Check sheet for the drawn part. Datum: minimum x, y, z corner. Units: mm. Coordinates: 2 decimals unless noted, no trailing zeros. Loops run counter-clockwise (first coordinate to the right, second up) from the corner with the lowest first, then second, coordinate; pieces in that order, holes last. Notation, with made-up numbers: (19, 14) -> (78, 14) arc R23 ccw to (78, 43) -> close; hole circle Ø5 at (85.25, 86). An arc over 180 degrees is marked (long way). Use CSV: the item, a comma, the result in double quotes. Start each with the question number.
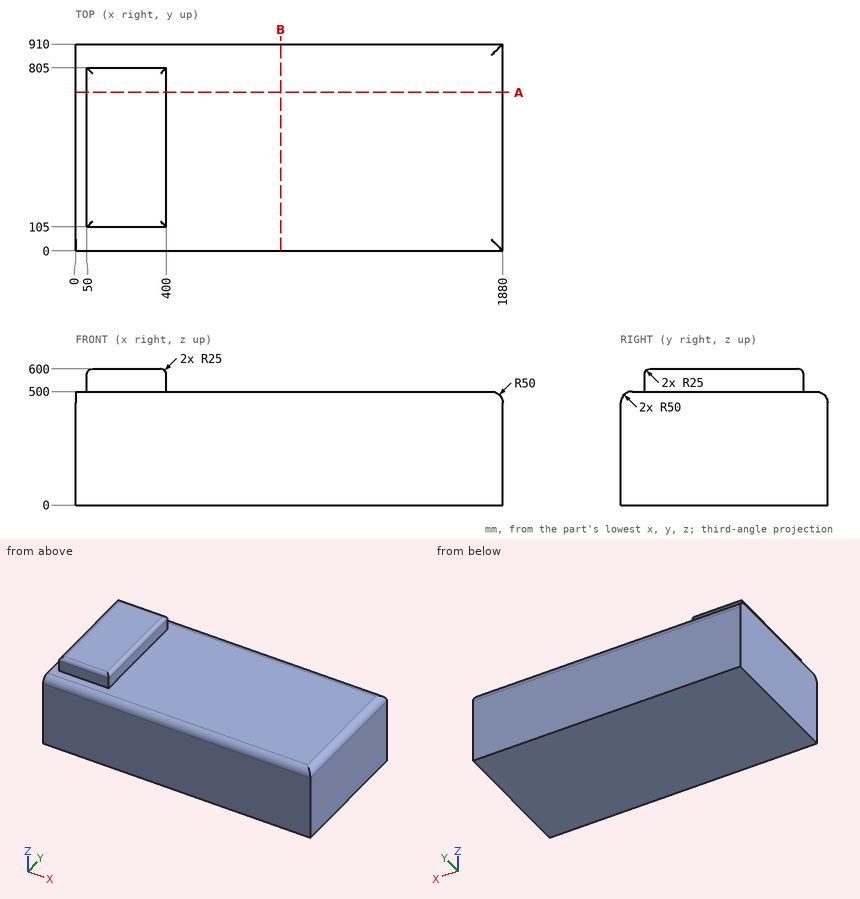
1. Depth check by flat-ended pin: pin 1 (1.5 mm diameter, centred on x = 1406, y = 538, fed in from +Z). Enter the tip coordinate at first touch or a pass-through.
2. Cross-section at A-A, the plane y = 697. Record the boundary of the cut face in (x, z).
3. Cross-section at B-B, the plane x = 903. Record the boundary of the cut face in (y, z).
4. Scan lines: line 1 (Z direction, x = 1678.5, y = 818.5); line 2 (X direction, y = 285.5, z = 538); line 3 (Y direction, x = 304.5, z = 518.5). Record each from-to range of solid material in increasing order.
Solution:
1,pin 1,"stops at z = 500"
2,outline,"(0, 0) -> (1880, 0) -> (1880, 450) arc R50 ccw to (1830, 500) -> (400, 500) -> (400, 575) arc R25 ccw to (375, 600) -> (75, 600) arc R25 ccw to (50, 575) -> (50, 500) -> (0, 500) -> close"
3,outline,"(0, 0) -> (910, 0) -> (910, 450) arc R50 ccw to (860, 500) -> (50, 500) arc R50 ccw to (0, 450) -> close"
4,line 1,"z = 0 to 500"
4,line 2,"x = 50 to 400"
4,line 3,"y = 105 to 805"
